from build123d import *

# Parameters (mm, degrees)
SKETCH2_R          = 13.335
EXTRUDE1_DEPTH     = 19.05
EXTRUDE1_DRAFT     = -1.5
EXTRUDE2_DEPTH     = 10.668
SKETCH4_OUTSIDE_W  = 249.236
SKETCH4_OUTSIDE_H  = 253.656
SKETCH4_OUTSIDE_R  = 14.2875
CUT_EXTRUDE1_DEPTH = 37.870978496
CUT_EXTRUDE1_DRAFT = -70
SKETCH23_OUTSIDE_W = 144.954
SKETCH23_OUTSIDE_H = 149.374
SKETCH23_OUTSIDE_R = 14.2875
CUT_EXTRUDE7_DEPTH = 29.969156551
CUT_EXTRUDE7_DRAFT = -60
SKETCH15_R         = 10.668
CUT_EXTRUDE2_DEPTH = 28.15732722
CUT_EXTRUDE2_DRAFT = -1.5
SKETCH17_R         = 9.307285714
CUT_EXTRUDE3_DEPTH = 28.15732722
SKETCH18_R         = 11.567261543
CUT_EXTRUDE6_DEPTH = 6.35
CUT_EXTRUDE6_DRAFT = -45


with BuildPart() as part:
    # Sketch2 → Extrude1 (with draft: the straight prism first)
    with BuildSketch(Plane(origin=(-9.525, 0, 0), x_dir=(0, 0, -1), z_dir=(1, 0, 0))):
        Circle(SKETCH2_R)
    extrude(amount=EXTRUDE1_DEPTH)
    # Extrude1: the draft: its side faces are tilted about the plane it starts from
    extrude1_sides = [part.faces().sort_by_distance(p)[0] for p in [
        (0, 0, 13.335),
    ]]
    draft(extrude1_sides, Plane(origin=(-9.525, 0, 0), x_dir=(0, 0, -1), z_dir=(1, 0, 0)), EXTRUDE1_DRAFT)

    # Sketch8 → Cut-Revolve1 (revolve, cut)
    with BuildSketch(Plane.XY, mode=Mode.PRIVATE) as cut_revolve1_sk:
        Polygon((-9.525, 14.281645334), (-9.525, 11.394586861), (-7.1024703, 14.281645334), align=None)
        Polygon((9.525, 12.528428667), (9.525, 14.281645334), (6.13892619, 14.281645334), (7.892142857, 12.528428667), align=None)
    revolve(cut_revolve1_sk.sketch.rotate(Axis((-9.525, 0, 0), (1, 0, 0)), 270), axis=Axis((-9.525, 0, 0), (1, 0, 0)), mode=Mode.SUBTRACT)

    # Sketch3 → Extrude2 (add)
    with BuildSketch(Plane(origin=(9.525, 0, 0), x_dir=(0, 0, -1), z_dir=(1, 0, 0))):
        Polygon((14.2875, 8.248891971), (0, 16.497783942), (-14.2875, 8.248891971), (-14.2875, -8.248891971), (0, -16.497783942), (14.2875, -8.248891971), align=None)
    extrude(amount=EXTRUDE2_DEPTH)


with BuildPart() as cut_extrude1_tool:
    # Sketch4 outside → Cut-Extrude1 (with draft: the straight prism first)
    with BuildSketch(Plane(origin=(20.193, 0, 0), x_dir=(0, 0, -1), z_dir=(1, 0, 0))):
        Rectangle(SKETCH4_OUTSIDE_W, SKETCH4_OUTSIDE_H)
        Circle(SKETCH4_OUTSIDE_R, mode=Mode.SUBTRACT)
    extrude(amount=-CUT_EXTRUDE1_DEPTH)
    # Cut-Extrude1: the draft: its side faces are tilted about the plane it starts from
    cut_extrude1_sides = [cut_extrude1_tool.faces().sort_by_distance(p)[0] for p in [
        (1.257510752, -126.828, 0),
        (1.257510752, 0, -124.618),
        (1.257510752, 126.828, 0),
        (1.257510752, 0, 124.618),
        (1.257510752, 0, 14.2875),
    ]]
    draft(cut_extrude1_sides, Plane(origin=(20.193, 0, 0), x_dir=(0, 0, -1), z_dir=(1, 0, 0)), CUT_EXTRUDE1_DRAFT)


with BuildPart() as part_1:
    add(part.part)

    # Cut-Extrude1: cut by cut_extrude1_tool
    add(cut_extrude1_tool.part, mode=Mode.SUBTRACT)


with BuildPart() as cut_extrude7_tool:
    # Sketch23 outside → Cut-Extrude7 (with draft: the straight prism first)
    with BuildSketch(Plane.ZY.offset(-9.525)):
        Rectangle(SKETCH23_OUTSIDE_W, SKETCH23_OUTSIDE_H)
        Circle(SKETCH23_OUTSIDE_R, mode=Mode.SUBTRACT)
    extrude(amount=-CUT_EXTRUDE7_DEPTH)
    # Cut-Extrude7: the draft: its side faces are tilted about the plane it starts from
    cut_extrude7_sides = [cut_extrude7_tool.faces().sort_by_distance(p)[0] for p in [
        (24.509578275, -74.687, 0),
        (24.509578275, 0, 72.477),
        (24.509578275, 74.687, 0),
        (24.509578275, 0, -72.477),
        (24.509578275, 0, -14.2875),
    ]]
    draft(cut_extrude7_sides, Plane.ZY.offset(-9.525), CUT_EXTRUDE7_DRAFT)


with BuildPart() as part_2:
    add(part_1.part)

    # Cut-Extrude7: cut by cut_extrude7_tool
    add(cut_extrude7_tool.part, mode=Mode.SUBTRACT)


with BuildPart() as cut_extrude2_tool:
    # Sketch15 → Cut-Extrude2 (with draft: the straight prism first)
    with BuildSketch(Plane(origin=(6.63702, 0, 0), x_dir=(0, 0, -1), z_dir=(1, 0, 0))):
        Circle(SKETCH15_R)
    extrude(amount=CUT_EXTRUDE2_DEPTH)
    # Cut-Extrude2: the draft: its side faces are tilted about the plane it starts from
    cut_extrude2_sides = [cut_extrude2_tool.faces().sort_by_distance(p)[0] for p in [
        (20.71568361, 0, 10.668),
    ]]
    draft(cut_extrude2_sides, Plane(origin=(6.63702, 0, 0), x_dir=(0, 0, -1), z_dir=(1, 0, 0)), CUT_EXTRUDE2_DRAFT)


with BuildPart() as part_3:
    add(part_2.part)

    # Cut-Extrude2: cut by cut_extrude2_tool
    add(cut_extrude2_tool.part, mode=Mode.SUBTRACT)

    # Sketch17 → Cut-Extrude3 (cut, through all)
    with BuildSketch(Plane(origin=(6.63702, 0, 0), x_dir=(0, 0, -1), z_dir=(1, 0, 0))):
        Circle(SKETCH17_R)
    extrude(amount=-CUT_EXTRUDE3_DEPTH, mode=Mode.SUBTRACT)


with BuildPart() as cut_extrude6_tool:
    # Sketch18 → Cut-Extrude6 (with draft: the straight prism first)
    with BuildSketch(Plane(origin=(20.193, 0, 0), x_dir=(0, 0, -1), z_dir=(1, 0, 0))):
        Circle(SKETCH18_R)
    extrude(amount=-CUT_EXTRUDE6_DEPTH)
    # Cut-Extrude6: the draft: its side faces are tilted about the plane it starts from
    cut_extrude6_sides = [cut_extrude6_tool.faces().sort_by_distance(p)[0] for p in [
        (17.018, 0, 11.567261543),
    ]]
    draft(cut_extrude6_sides, Plane(origin=(20.193, 0, 0), x_dir=(0, 0, -1), z_dir=(1, 0, 0)), CUT_EXTRUDE6_DRAFT)


with BuildPart() as part_4:
    add(part_3.part)

    # Cut-Extrude6: cut by cut_extrude6_tool
    add(cut_extrude6_tool.part, mode=Mode.SUBTRACT)


solid = part_4.part
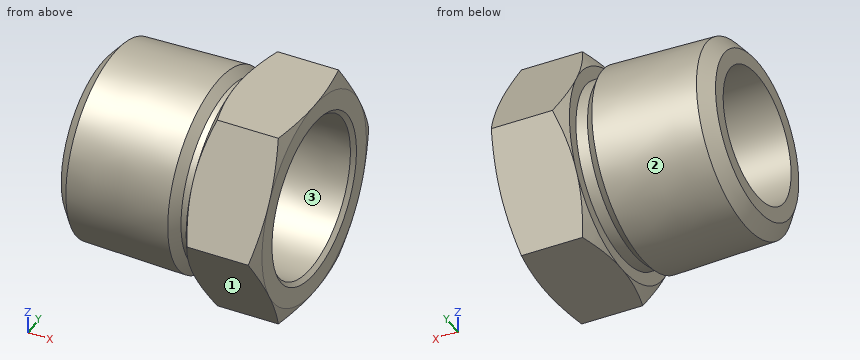
Design review of the part built by this model. Coordinates are the model's own, in mm. Face numbers are marked on the shaded views. Give positions to 0.01 mm unless a question says otherwise; leave off trailing zeros. Write each loop counter-clockwise with the first axis right and the second up, starting at its lowest first coordinate (ties: lowest second). Pieces come first, ordered by that corner, then holes. Notation, with made-up numbers: M 49.25,-40 L 69.25,-40 A30 cw 69.25,-12 Z; hole C 19.25,-18 d4. An arc over 180 degrees is marked long. Return JSON: item names as keys, results as strings. Group by question number.
Item 1: Clearance check with flat-ended pins moving along their axes: pin 1 Ø8 at (x, z) = (6, -7) entering from -Y; pin 2 Ø3 at (x, y) = (13.5, -10.5) entering from -Z; pin 3 Ø3 at (x, z) = (11, -8) entering from +Y (3 decimals). State where each tip first meets the part, or that it passes through.
Item 2: Take a section at B-B (x = -6.75). Give the boundary of the cut face in (y, z), plus the area to 3 significant figures.
Item 3: Take a section at A-A (x = 2.5). Give the boundary of the cut face in (y, z).
Item 4: Wall thickness on line 1 along Y through (x, z) = (6.25, -1.5); line 2 along Y through (x, z) = (-0.5, -4.75); line 3 along X through (y, z) = (-7, -10.5) (3 decimals): over which ranges is each line inside the solid? List them lowest first.
Item 5: The part is to be moulded in two halves that separate along Z. For the marked faces 1, 2 and 3, say which applies: pulls with the +Z half, pulls with the -Z half, needs draft (parallel to the pull), parting line crosses it, or undercut.
Return value:
{
 "1": {"pin 1": "stops at y = -13.44", "pin 2": "stops at z = -12.99", "pin 3": "stops at y = 12.745"},
 "2": {"outline": "C 0,0 d26.82; hole C 0,0 d18.61", "area": "293 mm2"},
 "3": {"outline": "C 0,0 d27.3; hole C 0,0 d18.61"},
 "4": {"line 1": "y = -13.67 to -9.19, 9.19 to 13.67", "line 2": "y = -12.71 to -8, 8 to 12.71", "line 3": "x = -8.497 to 7.801, 9.525 to 20.193"},
 "5": {"face 1": "pulls with the -Z half", "face 2": "parting line crosses it", "face 3": "undercut"}
}
